Build history of the part. All positions in model axes, mm. Face numbers are marked on the shaded views. Coordinates: 2 decimals unless noted, no trailing zeros. One line per item, written item: value.
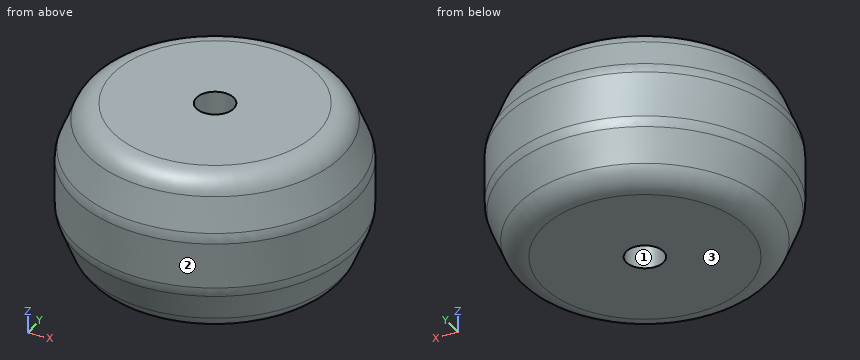
```python
from build123d import *

# Parameters (mm, degrees)
F0_R     = 9
F0_R_2   = 1.4
F1_DEPTH = 12
F4_R     = 2


with BuildPart() as f1:
    # F0 (on Top) → F1 (new body)
    with BuildSketch(Plane.XY):
        Circle(F0_R)
        Circle(F0_R_2, mode=Mode.SUBTRACT)
    extrude(amount=F1_DEPTH)

    # F2 (on Front) → F3 (revolve)
    with BuildSketch(Plane.XZ):
        Polygon((-10.558846, 3.9), (-9, 0), (-9, 12), (-10.558846, 8.1), align=None)
    revolve(axis=Axis((0, 0, 12), (0, 0, 1)))

    # F4
    f4_edges = [f1.edges().sort_by_distance(p)[0] for p in [
        (10.558846, 0, 3.9),
        (10.558846, 0, 8.1),
        (-9.779423, 0, 1.95),
        (9, 0, 0),
        (9, 0, 12),
    ]]
    fillet(f4_edges, radius=F4_R)


solid = f1.part
```
Item 1: Drop flat-ended pins along their axis: P1, Ø12, axis at x = 7, y = -4, coming from the +Z side; P2, Ø4, axis at y = -5, z = 10, coming from the -X side; P3, Ø1.5, axis at y = -0.5, z = 3, coming from the +X side; P4, Ø5, axis at x = -6.5, z = 2, coming from the +Y side. Give the stop position or say it passes through.
Check result:
P1: stops at z = 12
P2: stops at x = -9.73
P3: stops at x = 10.48
P4: stops at y = 9.38
Item 2: Probe probe 1 along Y at (x, z) = (0, 8.25); probe 2 along X at (y, z) = (-6.75, 9); probe 3 along Y at (x, z) = (0, 9.5). List the from-to ranges inside material, lowest first. Write a range as from..to.
Check result:
probe 1: y = -10.49..-1.4, 1.4..10.49
probe 2: x = -7.65..7.65
probe 3: y = -10..-1.4, 1.4..10
Item 3: Pull direction X, two halves, no side cores. Call the marked faces 1, 2 and 3: released by +X, released by -X, zero draft, split by the parting line, or undercut.
Check result:
face 1: undercut
face 2: split by the parting line
face 3: zero draft
